from build123d import *

# Parameters (mm, degrees)
F2_R = 9.525


with BuildPart() as f3:
    # F3: sweep along a path in F0
    with BuildLine(Plane.YZ) as f3_path:
        Line((0, 0), (0, 588.01))
        ThreePointArc((0, 588.01), (-6.3235645942, 603.2764354058), (-21.59, 609.6))
        Line((-21.59, 609.6), (-46.99, 609.6))
    # F2 (on offset) → F3 (sweep)
    with BuildSketch(Plane.XZ.offset(46.99)):
        with Locations((0, 609.6)):
            Circle(F2_R)
    sweep(path=f3_path.line)

    # F4: F3 across plane


with BuildPart() as f3_1:
    add(f3.part)
    add(f3.part.mirror(Plane.XY))


solid = f3_1.part
Model file for the job. Use its own axes, mm. A direction names the side the tool comes from. Give positions to 0.01 mm unless a question says otherwise; leave off trailing zeros. Loops run counter-clockwise (first coordinate to the right, second up) from the corner with the lowest first, then second, coordinate; pieces in that order, holes last. Notation, with made-up numbers: (0.25, 25.25) -> (17.25, 25.25) arc R21 cw to (17.25, 45.25) -> close; hole circle Ø6 at (12.25, 68.5). An arc over 180 degrees is marked (long way). Use a Markdown table: item, result. Add a question column.
(1) Slice it at C-C on z = -391.5. List the corners of the cut face in (x, y) (3 decimals), and give its area (3 significant figures).
(2) Slice it at A-A on x = 0. List the corners of the cut face in (y, z) (3 decimals), and give its area (3 significant figures).
(3) Slice it at B-B on y = -37. List the corners of the cut face in (x, z) (3 decimals), and give its area (3 significant figures).
(4) Drop flat-ended pins along their axis: pin 1 Ø4 at (x, y) = (-2.5, -35.5) entering from +Z; pin 2 Ø1 at (x, y) = (1, 2) entering from +Z; pin 3 Ø4 at (x, z) = (3, -152) entering from +Y. Give the stop position or say it passes through.
(5) Mould opens along Z. For faces 1 (the cylindrical face through (-7.02, -34.47, -616.04)), 2 (the flat face through (0, -46.99, 610)) say: +Z half, -Z half, draft (parallel to the pull), parting line (faces both ways), or undercut.
(6) Wall check: line 1 along Z through (x, y) = (-0.5, -36.5); line 2 along Y through (x, z) = (2, 545.5); line 3 along Z through (x, y) = (-7, -41.5). Give the ranges that are in metal, low to high.
(7) Tool access for faces 3 (the cylindrical face through (-7.02, -34.47, 616.04)), 4 (the flat face through (0, -46.99, -610)): list every direction of +Z, -Z, +X, -X, +Y, -Y with a clear straight run to the whole face (end or side of a thin tool).
Filled sheet:
| question | item | result |
|---|---|---|
| 1 | outline | circle Ø19.05 at (0, 0) |
| 1 | area | 285 mm2 |
| 2 | outline | (-46.99, -619.125) -> (-21.59, -619.125) arc R31.115 ccw to (9.525, -588.01) -> (9.525, 588.01) arc R31.115 ccw to (-21.59, 619.125) -> (-46.99, 619.125) -> (-46.99, 600.075) -> (-21.59, 600.075) arc R12.065 cw to (-9.525, 588.01) -> (-9.525, -588.01) arc R12.065 cw to (-21.59, -600.075) -> (-46.99, -600.075) -> close |
| 2 | area | 24,700 mm2 |
| 3 | outline | circle Ø19.05 at (0, -609.6); circle Ø19.05 at (0, 609.6) |
| 3 | area | 570 mm2 |
| 4 | pin 1 | z = 619.11 |
| 4 | pin 2 | z = 608.79 |
| 4 | pin 3 | y = 9.47 |
| 5 | face 1 | undercut |
| 5 | face 2 | draft |
| 6 | line 1 | -619.11 to -600.09, 600.09 to 619.11 |
| 6 | line 2 | -9.31 to 9.31 |
| 6 | line 3 | -616.06 to -603.14, 603.14 to 616.06 |
| 7 | face 3 | -Y |
| 7 | face 4 | +Z, -Z, +X, -X, -Y |
